Read the model definition and answer for the solid it produces. Units are mm, in the model's axes. Face numbers are marked on the shaded views. A direction names the side the tool comes from. Round coordinates to 2 decimals unless told otherwise and drop trailing zeros. Write each loop counter-clockwise with the first axis right and the second up, starting at its lowest first coordinate (ties: lowest second). Pieces come first, ordered by that corner, then holes. Notation, with made-up numbers: (34.25, -2) - (63.25, -2) arc R24 cw to (63.25, 25) - close; hole circle Ø9 at (29, -29.75). An arc over 180 degrees is marked (long way). Use one line per item in the form item = value. Start each with the question number.
1) For a pull along X with two mould halves and no side action, classify the marked faces 1, 2 and 3 as released by +X, released by -X, zero draft, split by the parting line, or undercut.
2) The part is cut by section A-A, the plane z = 0. Give the vertices of the cut face in (x, y), plus the area to 3 significant figures.
3) The part is cut by section B-B, the plane y = -25. Give the vertices of the cut face in (x, z).
4) Each of these flat-tipped pins is pushed along its axis until it touches: pin 1 (2 mm diameter, centred on y = -10.5, z = 1.5, fed in from +X); pin 2 (1.5 mm diameter, centred on y = -8, z = -2, fed in from -X); pin 3 (5 mm diameter, centred on x = 3, y = -18, fed in from +Z). Where does it stop, or does it pass through?
5) For the marked faces 4, 5 and 6, determine the directions among +Z, -Z, +X, -X, +Y, -Y from which every point of the face is accessible in a straight line to the end or side of a thin tool.
6) Consider line 1 along Y through (x, z) = (-3.25, 1); line 2 along Y through (x, z) = (-2.25, 1); line 3 along X through (y, z) = (-6, 1.5). Determine where each line is inside the solid, lowest interval first. Write a range as from..to.
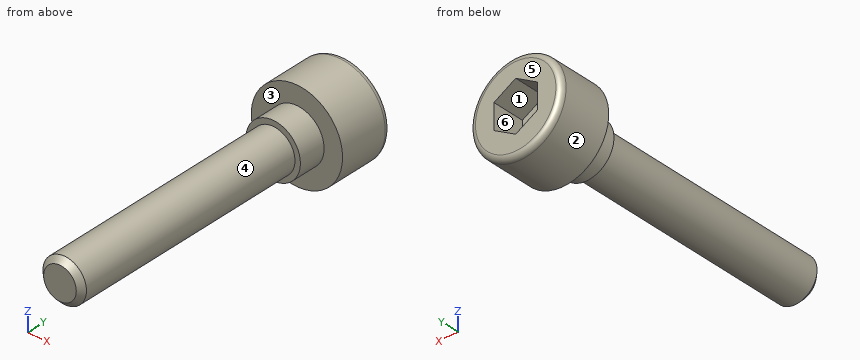
from build123d import *

# Parameters (mm, degrees)
CORTAR_EXTRUIR1_DEPTH = 3
CHAFL_N1_SIZE         = 0.5
REDONDEO1_R           = 0.5
CROQUIS3_W            = 0.5
CROQUIS3_H            = 22.5
CHAFL_N2_SIZE         = 0.5


with BuildPart() as part:
    # Croquis1 → Revolución1 (revolve)
    with BuildSketch(Plane.XY):
        Polygon((0, 0), (4.2, 0), (4.2, -5), (2.5, -5), (2.5, -30), (0, -30), align=None)
    revolve(axis=Axis((0, 0, 0), (0, -1, 0)))

    # Croquis2 → Cortar-Extruir1 (cut)
    with BuildSketch(Plane(origin=(0, 0, 0), x_dir=(1, 0, 0), z_dir=(0, 1, 0))):
        Polygon((2, 1.154700538), (0, 2.309401077), (-2, 1.154700538), (-2, -1.154700538), (0, -2.309401077), (2, -1.154700538), align=None)
    extrude(amount=-CORTAR_EXTRUIR1_DEPTH, mode=Mode.SUBTRACT)

    # Chaflán1
    chafl_n1_edges = [part.edges().sort_by_distance(p)[0] for p in [
        (-2.5, -30, 0),
    ]]
    chamfer(chafl_n1_edges, length=CHAFL_N1_SIZE)

    # Redondeo1
    redondeo1_edges = [part.edges().sort_by_distance(p)[0] for p in [
        (-4.2, 0, 0),
    ]]
    fillet(redondeo1_edges, radius=REDONDEO1_R)

    # Croquis3 → Cortar-Revolución1 (revolve, cut)
    with BuildSketch(Plane.XY):
        with Locations((2.25, -18.75)):
            Rectangle(CROQUIS3_W, CROQUIS3_H)
    revolve(axis=Axis((0, 0, 0), (0, -1, 0)), mode=Mode.SUBTRACT)

    # Chaflán2
    chafl_n2_edges = [part.edges().sort_by_distance(p)[0] for p in [
        (-2, -30, 0),
    ]]
    chamfer(chafl_n2_edges, length=CHAFL_N2_SIZE)


solid = part.part
Geometry results:
q1.face_1 = undercut
q1.face_2 = split by the parting line
q1.face_3 = zero draft
q2.outline = (-4.2, -5) - (-2.5, -5) - (-2.5, -7.5) - (-2, -7.5) - (-2, -29.5) - (-1.5, -30) - (1.5, -30) - (2, -29.5) - (2, -7.5) - (2.5, -7.5) - (2.5, -5) - (4.2, -5) - (4.2, -0.5) arc R0.5 ccw to (3.7, 0) - (2, 0) - (2, -3) - (-2, -3) - (-2, 0) - (-3.7, 0) arc R0.5 ccw to (-4.2, -0.5) - close
q2.area = 132 mm2
q3.outline = circle Ø4 at (0, 0)
q4.pin_1 = 1.94
q4.pin_2 = -2.04
q4.pin_3 = 1.94
q5.face_4 = -Y
q5.face_5 = +Z, -Z, +X, -X, +Y
q5.face_6 = +Y
q6.line_1 = -5..0
q6.line_2 = -7.5..0
q6.line_3 = -2..2
